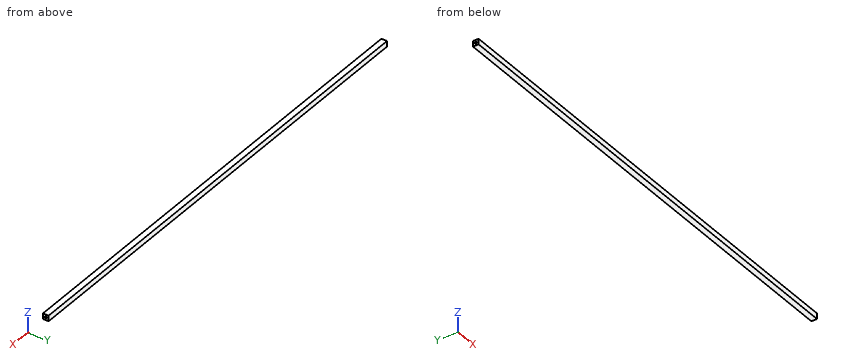
```python
from build123d import *

# Parameters (mm, degrees)
F0_W     = 1270
F0_H     = 15
F1_DEPTH = 7.5
F2_W     = 5
F2_H     = 5
F3_DEPTH = 190.5
F4_DEPTH = 1270


with BuildPart() as f1:
    # F0 (on Front) → F1 (new body, symmetric)
    with BuildSketch(Plane.XZ):
        with Locations((-3.320781514, -27.9977901512)):
            Rectangle(F0_W, F0_H)
    extrude(amount=F1_DEPTH, both=True)

    # F2 (on face) → F3 (cut, symmetric)
    with BuildSketch(Plane.YZ.offset(631.679218486)):
        with Locations((0, -27.9977901512)):
            Rectangle(F2_W, F2_H)
    extrude(amount=F3_DEPTH, both=True, mode=Mode.SUBTRACT)

    # F4 (cut): a face of the model
    f4_faces = [f1.faces().sort_by_distance(p)[0] for p in [
        (441.179218486, 0, -27.9977901512),
    ]]
    extrude(f4_faces, amount=-F4_DEPTH, mode=Mode.SUBTRACT)


solid = f1.part
```
For this review, take the finished solid that the model builds, in its own axes (mm). Round coordinates to 2 decimals unless told otherwise and drop trailing zeros. Write each loop counter-clockwise with the first axis right and the second up, starting at its lowest first coordinate (ties: lowest second). Pieces come first, ordered by that corner, then holes. Notation, with made-up numbers: (-37, 42) -> (-2, 42) arc R26 ccw to (-2, 67) -> close; hole circle Ø5 at (54.25, 81.5). An arc over 180 degrees is marked (long way). Use one line per item in the form item = value.
1) Take a section at A-A, the plane y = -0.25. Write out the cut boundary in (x, z), and give its area (3 significant figures).
Found:
outline = (-638.32, -35.5) -> (631.68, -35.5) -> (631.68, -30.5) -> (-638.32, -30.5) -> close; (-638.32, -25.5) -> (631.68, -25.5) -> (631.68, -20.5) -> (-638.32, -20.5) -> close
area = 12,700 mm2
2) To check wall thickness, follow L1, parallel to Z at x = 312, y = -2; L2, parallel to Y at x = 276, z = -29.5. State the ranges of each line that lie inside material, in increasing order. Write a range as from..to.
Found:
L1 = -35.5..-30.5, -25.5..-20.5
L2 = -7.5..-2.5, 2.5..7.5
3) Take a section at B-B, the plane x = 276. Write out the cut boundary in (y, z).
Found:
outline = (-7.5, -35.5) -> (7.5, -35.5) -> (7.5, -20.5) -> (-7.5, -20.5) -> close; hole (-2.5, -30.5) -> (2.5, -30.5) -> (2.5, -25.5) -> (-2.5, -25.5) -> close
